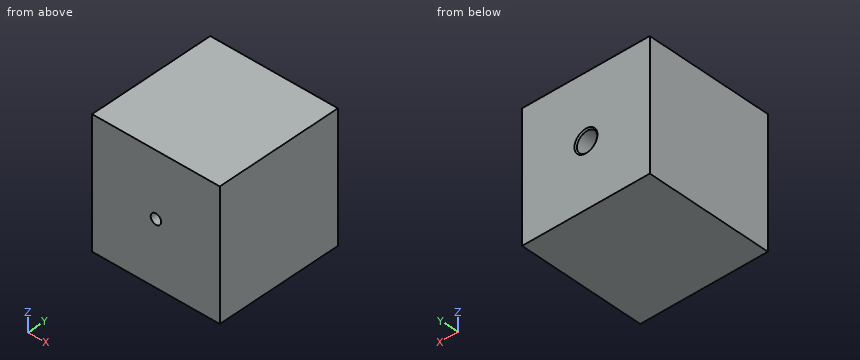
from build123d import *

# Parameters (mm, degrees)
SKICA1_W                 = 50
SKICA1_H                 = 50
P_IDAT_VYSUNUT_M1_DEPTH  = 50
SKICA2_R                 = 2.05
ODEBRAT_VYSUNUT_M1_DEPTH = 50
SKICA3_R                 = 4
ODEBRAT_VYSUNUT_M2_DEPTH = 25
ZKOSEN_1_SIZE            = 0.5
ZKOSEN_2_SIZE            = 0.5


with BuildPart() as part:
    # Skica1 → Přidat vysunutím1 (new body)
    with BuildSketch(Plane.XY):
        Rectangle(SKICA1_W, SKICA1_H)
    extrude(amount=P_IDAT_VYSUNUT_M1_DEPTH)

    # Skica2 → Odebrat vysunutím1 (cut)
    with BuildSketch(Plane(origin=(0, 25, 0), x_dir=(1, 0, 0), z_dir=(0, 1, 0))):
        with Locations(Location((0, -25, 0), (0, 0, 270))):
            Circle(SKICA2_R)
    extrude(amount=-ODEBRAT_VYSUNUT_M1_DEPTH, mode=Mode.SUBTRACT)

    # Skica3 → Odebrat vysunutím2 (cut)
    with BuildSketch(Plane(origin=(0, 25, 0), x_dir=(1, 0, 0), z_dir=(0, 1, 0))):
        with Locations(Location((0, -25, 0), (0, 0, 270))):
            Circle(SKICA3_R)
    extrude(amount=-ODEBRAT_VYSUNUT_M2_DEPTH, mode=Mode.SUBTRACT)

    # Zkosení1
    zkosen_1_edges = [part.edges().sort_by_distance(p)[0] for p in [
        (0, 25, 21),
    ]]
    chamfer(zkosen_1_edges, length=ZKOSEN_1_SIZE)

    # Zkosení2
    zkosen_2_edges = [part.edges().sort_by_distance(p)[0] for p in [
        (0, 0, 22.95),
    ]]
    chamfer(zkosen_2_edges, length=ZKOSEN_2_SIZE)


solid = part.part
CAD build for the part. Positions are in the model's coordinates, mm. Coordinates: 2 decimals unless noted, no trailing zeros. Loops run counter-clockwise (first coordinate to the right, second up) from the corner with the lowest first, then second, coordinate; pieces in that order, holes last. Notation, with made-up numbers: (73.5, 35) - (101.5, 35) arc R3 ccw to (101.5, 40) - close; hole circle Ø10 at (-2, -30.5). An arc over 180 degrees is marked (long way). Use one line per item in the form item = value. Start each with the question number.
1) Flat gauge pin, fed straight in: pin 1 (3.5 mm diameter, centred on x = 0, z = 25, fed in from -Y). Where does the tip first touch, or does it go through?
2) Band-saw the part on B-B (x = 0). Give the cut face in (y, z).
3) Band-saw the part on A-A (z = 25). Give the cut face in (x, y).
4) Drill centre lines: L1, parallel to X at y = -13, z = 25; L2, parallel to X at y = 13, z = 25; L3, parallel to Z at x = -0.5, y = -11. Where is each one in solid material? Low to high. Write a range as from..to.
Check values:
q1.pin_1 = through
q2.outline = (-25, 0) - (25, 0) - (25, 20.5) - (24.5, 21) - (0, 21) - (0, 22.45) - (-0.5, 22.95) - (-25, 22.95) - close; (-25, 27.05) - (-0.5, 27.05) - (0, 27.55) - (0, 29) - (24.5, 29) - (25, 29.5) - (25, 50) - (-25, 50) - close
q3.outline = (-25, -25) - (-2.05, -25) - (-2.05, -0.5) - (-2.55, 0) - (-4, 0) - (-4, 24.5) - (-4.5, 25) - (-25, 25) - close; (2.05, -25) - (25, -25) - (25, 25) - (4.5, 25) - (4, 24.5) - (4, 0) - (2.55, 0) - (2.05, -0.5) - close
q4.L1 = -25..-2.05, 2.05..25
q4.L2 = -25..-4, 4..25
q4.L3 = 0..23.01, 26.99..50
